Print and shaded views of the part. All mm, measured from the part's lowest x, y and z. A direction names the side the tool comes from. Round coordinates to 2 decimals unless told otherwise and drop trailing zeros. Write each loop counter-clockwise with the first axis right and the second up, starting at its lowest first coordinate (ties: lowest second). Pieces come first, ordered by that corner, then holes. Notation, with made-up numbers: (0, 20) - (17, 20) arc R26 cw to (17, 49) - close; hole circle Ø11 at (42, 77.25). An arc over 180 degrees is marked (long way). Answer as a JSON object with one key per item and string values. Group by question number.
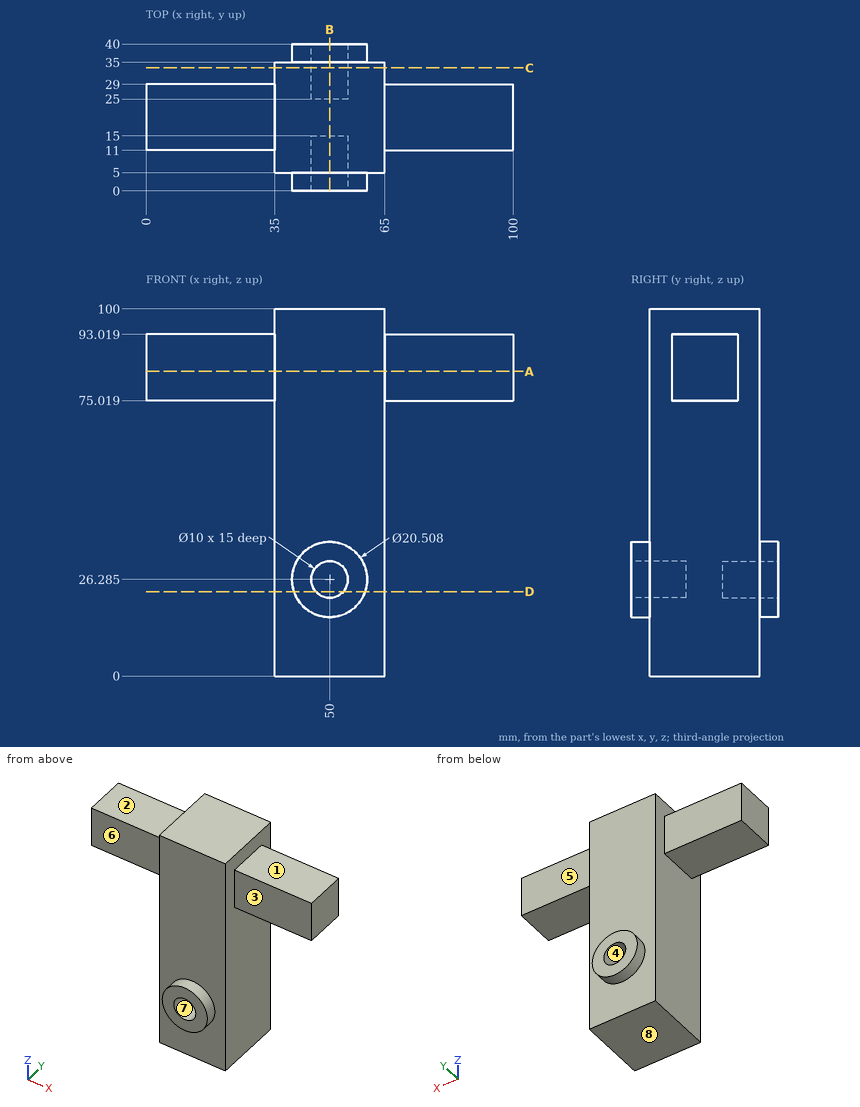
(1) Pull direction Z, two halves, no side cores. Call the marked faces 6, 7 and 8: pulls with the +Z half, pulls with the -Z half, needs draft (parallel to the pull), parting line crosses it, or undercut.
(2) Slice it at B-B (x = 50). Write the cut outline in (y, z) (1 decimal).
(3) Drill centre lines: line 1 (Z direction, x = 50, y = 28.75) (1 decimal); line 2 (X direction, y = 30, z = 81.5); line 3 (Y direction, x = 62, z = 64). Where is each one in solid material? Low to high. Write a range as from..to.
(4) 3-axis set-ups, long thin cutter, end or side, ignore diameter. For the marked faces 1, 2, 3, 4 and 5: which of +Z, -Z, +X, -X, +Y, -Y reach the whole face in a straight line?
(5) Slice it at A-A (z = 83). Write the cut outline in (x, y).
(6) Slice it at D-D (z = 23). Write the cut outline in (x, y), then the cut area to 3 significant figures.
(7) Slice it at C-C (y = 33.5). Write the cut outline in (x, z) (1 decimal), then the cut area to 3 significant figures.
(8) Flat gauge pins, fed straight in: pin 1 (14.5 mm diameter, centred on x = 80.5, y = 16.5, fed in from +Z); pin 2 (20 mm diameter, centred on x = 85, z = 82, fed in from -Y); pin 3 (2 mm diameter, centred on y = 4.5, z = 77.5, fed in from +X). Where does each tip first touch, or does it go through?
Answer:
{
 "1": {"face 6": "needs draft", "face 7": "undercut", "face 8": "pulls with the -Z half"},
 "2": {"outline": "(0, 16) - (5, 16) - (5, 0) - (35, 0) - (35, 16) - (40, 16) - (40, 21.3) - (25, 21.3) - (25, 31.3) - (40, 31.3) - (40, 36.5) - (35, 36.5) - (35, 100) - (5, 100) - (5, 36.5) - (0, 36.5) - (0, 31.3) - (15, 31.3) - (15, 21.3) - (0, 21.3) - close"},
 "3": {"line 1": "0..21.3, 31.3..100", "line 2": "35..65", "line 3": "5..35"},
 "4": {"face 1": "+Z, +X, +Y, -Y", "face 2": "+Z, -X, +Y, -Y", "face 3": "+Z, -Z, +X, -Y", "face 4": "+Y", "face 5": "+Z, -Z, +X, +Y"},
 "5": {"outline": "(0, 11) - (35, 11) - (35, 5) - (65, 5) - (65, 11) - (100, 11) - (100, 29) - (65, 29) - (65, 35) - (35, 35) - (35, 29) - (0, 29) - close"},
 "6": {"outline": "(35, 5) - (40.29, 5) - (40.29, 0) - (46.23, 0) - (46.23, 15) - (53.77, 15) - (53.77, 0) - (59.71, 0) - (59.71, 5) - (65, 5) - (65, 35) - (59.71, 35) - (59.71, 40) - (53.77, 40) - (53.77, 25) - (46.23, 25) - (46.23, 40) - (40.29, 40) - (40.29, 35) - (35, 35) - close", "area": "868 mm²"},
 "7": {"outline": "(35, 0) - (65, 0) - (65, 100) - (35, 100) - close; hole circle Ø10 at (50, 26.3)", "area": "2,920 mm²"},
 "8": {"pin 1": "z = 93.02", "pin 2": "y = 11", "pin 3": "x = 65"}
}
